from build123d import *

# Parameters (mm, degrees)
SKETCH1_W           = 6.35
SKETCH1_H           = 48.26
BOSS_EXTRUDE1_DEPTH = 3.175
SKETCH3_R           = 1.4605
CUT_EXTRUDE2_DEPTH  = 4.175
BOSS_EXTRUDE3_DEPTH = 3.175


with BuildPart() as part:
    # Sketch1 → Boss-Extrude1 (new body)
    with BuildSketch(Plane.XY):
        with Locations((3.175, 24.13)):
            Rectangle(SKETCH1_W, SKETCH1_H)
    extrude(amount=BOSS_EXTRUDE1_DEPTH)

    # Sketch3 → Cut-Extrude2 (cut, through all)
    with BuildSketch(Plane.XY.offset(3.175)):
        with Locations((3.175, 43.18)):
            Circle(SKETCH3_R)
    extrude(amount=-CUT_EXTRUDE2_DEPTH, mode=Mode.SUBTRACT)

    # Sketch5 → Boss-Extrude3 (add)
    with BuildSketch(Plane(origin=(0, 0, 0), x_dir=(-1, 0, 0), z_dir=(0, 0, -1))):
        Polygon((-6.35, 12.7), (-16.51, 12.7), (-16.51, 0), (-11.43, 0), (-11.43, 7.62), (-6.35, 7.62), align=None)
    extrude(amount=-BOSS_EXTRUDE3_DEPTH)


solid = part.part
The listing builds one solid part. Answer for the finished solid, in the listing's coordinates (mm). A direction names the side the tool comes from. Round coordinates to 2 decimals unless told otherwise and drop trailing zeros. Order: outer loops, then holes, each group sorted by start corner. A loop starts at its lowest first (then second) coordinate and runs counter-clockwise, first axis right, second up. Notation, with made-up numbers: (24.5, -8) -> (32.5, -8) arc R19 cw to (32.5, 13) -> close; hole circle Ø5 at (26, 19). An arc over 180 degrees is marked (long way). One line per item, written item: value.
Item 1: Find section C-C, the plane x = 2.5. Give the vertices of the cut face in (y, z) (3 decimals), then the cut area to 3 significant figures.
Taken from the geometry:
outline: (0, 0) -> (41.885, 0) -> (41.885, 3.175) -> (0, 3.175) -> close; (44.475, 0) -> (48.26, 0) -> (48.26, 3.175) -> (44.475, 3.175) -> close
area: 145 mm2
Item 2: For faces 1 (the flat face through (6.35, 4, 2)), 2 (the flat face through (11, 12.7, 2)), 3 (the flat face through (3, 48.26, 2)), determine the directions among +Z, -Z, +X, -X, +Y, -Y from which every point of the face is accessible in a straight line to the end or side of a thin tool.
Taken from the geometry:
face 1: +Z, -Z, -Y
face 2: +Z, -Z, +X, +Y
face 3: +Z, -Z, +X, -X, +Y
Item 3: For a pull along Y with two mould halves and no side action, classify faces 4 (the flat face through (16.51, 6, 2)), 5 (the cylindrical face through (3.96, 44.41, 1.61)), 6 (the flat face through (14, 0, 2)) as released by +Y, released by -Y, zero draft, split by the parting line, or undercut.
Taken from the geometry:
face 4: zero draft
face 5: undercut
face 6: released by -Y
Item 4: Find section D-D, the plane y = 36. Give the vertices of the cut face in (x, z) (3 decimals), then the cut area to 3 significant figures.
Taken from the geometry:
outline: (0, 0) -> (6.35, 0) -> (6.35, 3.175) -> (0, 3.175) -> close
area: 20.2 mm2
Item 5: Straight lines are drawn through the part: L1, parallel to X at y = 6.5, z = 2.2; L2, parallel to X at y = 43.5, z = 1.75; L3, parallel to X at y = 36, z = 1.4. For each, find the intervals that lie inside material, in ascending order.
Taken from the geometry:
L1: x = 0 to 6.35, 11.43 to 16.51
L2: x = 0 to 1.75, 4.6 to 6.35
L3: x = 0 to 6.35
Item 6: Given P1, Ø1, axis at y = 32, z = 2.5, coming from the +X side, flat-ended and moving along its own axis, determine where the tip first touches the part or whether it passes through.
Taken from the geometry:
P1: stops at x = 6.35
